Autodesk Inventor part; units mm, degrees
ref_plane "YZ Plane" through (0, 0, 0) normal (1, 0, 0) x (0, 1, 0)
ref_plane "XZ Plane" through (0, 0, 0) normal (0, 1, 0) x (-1, 0, 0)
ref_plane "XY Plane" through (0, 0, 0) normal (0, 0, 1) x (1, 0, 0)
sketch "Sketch1" plane through (0, 0, 0) normal (0, 1, 0) x (-1, 0, 0)
  line L0 (0, 0) -> (28, 0)
  line L1 (28, 0) -> (28, -38.5)
  line L2 (28, -38.5) -> (0, -38.5)
  line L3 (0, -38.5) -> (0, 0)
  dimension "d0" = 28
  dimension "d1" = 38.5
extrude "Extrusion1" add sketch "Sketch1" along normal blind 3
sketch "Sketch2" plane through (0, 3, 0) normal (0, 1, 0) x (1, 0, 0)
  line L0 (-28, 0) -> (0, 0)
  circle A0 centre (0, 0) radius 2
  circle A1 centre (-28, 0) radius 2
  line L1 (0, 38.5) -> (-28, 38.5)
  circle A2 centre (-28, 38.5) radius 2
  circle A3 centre (0, 38.5) radius 2
  dimension "d8" = 4
  dimension "d9" = 4
  dimension "d10" = 4
  dimension "d11" = 4
extrude "Extrusion2" cut sketch "Sketch2" against normal blind 3
sketch "Sketch3" plane through (0, 3, 0) normal (0, 1, 0) x (1, 0, 0)
  line L0 (-32.85, 43.35) -> (4.85, 43.35)
  line L1 (4.85, 43.35) -> (4.85, -4.85)
  line L2 (4.85, -4.85) -> (-32.85, -4.85)
  line L3 (-32.85, -4.85) -> (-32.85, 43.35)
  line L4 (-2, 38.5) -> (-26, 38.5)
  line L5 (0, 2) -> (0, 36.5)
  point P0 (0, 0)
  point P1 (-2, 6.25)
  point P2 (-26, 32.25)
  dimension "d14" = 48.2
  dimension "d15" = 37.7
  dimension "d16" = 4.85
  dimension "d17" = 4.85
extrude "Extrusion3" add sketch "Sketch3" along normal blind 2
sketch "Sketch4" plane through (0, 3, 0) normal (0, -1, 0) x (1, 0, 0)
  circle A0 centre (2.35, -40.85) radius 2.25
  line L0 (-2, -38.5) -> (-26, -38.5)
  line L1 (0, -2) -> (0, -36.5)
  circle A1 centre (-30.35, -40.85) radius 2.25
  line L2 (-28, -36.5) -> (-28, -2)
  circle A2 centre (-30.35, 2.35) radius 2.25
  line L3 (-26, 0) -> (-2, 0)
  circle A3 centre (2.35, 2.35) radius 2.25
  point P0 (0, 0)
  dimension "d20" = 4.5
  dimension "d21" = 2.35
  dimension "d22" = 2.35
  dimension "d23" = 4.5
  dimension "d24" = 2.35
  dimension "d25" = 2.35
  dimension "d26" = 4.5
  dimension "d27" = 2.35
  dimension "d28" = 4.5
  dimension "d29" = 2.35
  dimension "d30" = 2.35
  dimension "d31" = 2.35
extrude "Extrusion4" add sketch "Sketch4" along normal blind 3
fillet "Fillet1" radius 2 4 edges at (4.85, 4, -43.35) (4.85, 4, 4.85) (-32.85, 4, 4.85) (-32.85, 4, -43.35)
sketch "Sketch5" plane through (0, 5, 0) normal (0, 1, 0) x (1, 0, 0)
  circle A0 centre (0, 19.25) radius 1
  circle A1 centre (-28, 19.25) radius 1
  line L0 (4.85, -2.85) -> (4.85, 41.35)
  line L1 (-30.85, -4.85) -> (2.85, -4.85)
  point P0 (0, 0)
  dimension "d45" = 2
  dimension "d46" = 2
  dimension "d73" = 28
  dimension "d81" = 24.1
  dimension "d82" = 4.85
extrude "Extrusion6" cut sketch "Sketch5" against normal through all
sketch "Sketch8" plane through (0, 5, 0) normal (0, 1, 0) x (1, 0, 0)
  circle A0 centre (-14, 3.125) radius 2.5
  line L0 (-2, 6.25) -> (-26, 6.25)
  line L1 (-26, 0) -> (-2, 0)
  line L2 (-32.85, 41.35) -> (-32.85, -2.85)
  point P0 (0, 0)
  dimension "d68" = 5
  dimension "d69" = 3.125
  dimension "d70" = 18.85
extrude "Extrusion9" cut sketch "Sketch8" against normal through all
sketch "Sketch10" plane through (0, 5, 0) normal (0, 1, 0) x (1, 0, 0)
  line L0 (-25.5, 12.75) -> (-2.5, 12.75)
  line L1 (-2.5, 12.75) -> (-2.5, 25.75)
  line L2 (-2.5, 25.75) -> (-25.5, 25.75)
  line L3 (-25.5, 25.75) -> (-25.5, 12.75)
  line L4 (-32.85, 41.35) -> (-32.85, -2.85)
  circle A0 centre (-28, 19.25) radius 1
  point P0 (0, 0)
  dimension "d83" = 23
  dimension "d84" = 13
  dimension "d85" = 7.35
  dimension "d86" = 6.5
extrude "Extrusion11" cut sketch "Sketch10" against normal through all contours L3 L2 L1 L0
sketch "Sketch11" plane through (0, 5, 0) normal (0, 1, 0) x (1, 0, 0)
  line L0 (-32.85, 41.35) -> (-32.85, -2.85)
  line L1 (-32.85, 12.75) -> (4.85, 12.75)
  line L2 (4.85, 12.75) -> (4.85, 43.35)
  line L3 (4.85, 43.35) -> (-32.85, 43.35)
  line L4 (-32.85, 43.35) -> (-32.85, 12.75)
  line L5 (-2.5, 12.75) -> (-25.5, 12.75)
  point P0 (0, 0)
  point P1 (-30.85, 43.35)
  point P2 (4.85, 41.35)
extrude "Extrusion12" cut sketch "Sketch11" against normal through all
sketch "Sketch9" plane through (0, 5, 0) normal (0, 1, 0) x (1, 0, 0)
  circle A0 centre (-14, 3.125) radius 2.5
  line L0 (-15.5, 5.125) -> (-15.5, 12.75)
  line L1 (-15.5, 12.75) -> (-12.5, 12.75)
  line L2 (-12.5, 12.75) -> (-12.5, 5.125)
  arc A1 (-12.5, 5.125) -> (-15.5, 5.125) centre (-14, 3.125) ccw
  line L3 (4.85, 12.75) -> (-32.85, 12.75)
  point P0 (0, 0)
  point P1 (-14, 12.75)
  point P2 (-14, 12.75)
  dimension "d76" = 3
  dimension "d77" = 1.5
extrude "Extrusion13" cut sketch "Sketch9" against normal through all contours A0 L0 L1 L2
fillet "Fillet3" radius 2 2 edges at (-15.5, 2.5, -5.125) (-12.5, 2.5, -5.125)
sketch "Sketch12" plane through (2.35, 0, 2.35) normal (0, -1, 0) x (1, 0, 0)
  point P0 (-2.35, -2.35)
sketch "Sketch13" plane through (0, 5, 0) normal (0, 1, 0) x (1, 0, 0)
  circle A0 centre (2.35, -2.35) radius 2.25
  circle A1 centre (2.35, -2.35) radius 1.15
  circle A2 centre (-30.35, -2.35) radius 2.25
  circle A3 centre (-30.35, -2.35) radius 1.15
  point P0 (0, 0)
  dimension "d96" = 2.3
  dimension "d97" = 2.3
extrude "Extrusion14" cut sketch "Sketch13" against normal through all contours A1 | A3
sketch "Sketch15" plane through (0, 0, -12.75) normal (0, 0, -1) x (-1, 0, 0)
  line L0 (0, 3) -> (-4.85, 3)
  line L1 (30.85, 5) -> (-2.85, 5)
  line L2 (-4.85, 3) -> (2.5, 3)
  line L3 (2.5, 3) -> (2.5, 5)
  line L4 (2.5, 5) -> (-4.85, 5)
  line L5 (-4.85, 5) -> (-4.85, 3)
  line L6 (32.85, 5) -> (32.85, 3)
  line L7 (32.85, 5) -> (25.5, 5)
  line L8 (25.5, 5) -> (25.5, 3)
  line L9 (25.5, 3) -> (32.85, 3)
  line L10 (32.85, 3) -> (32.85, 5)
  point P0 (0, 0)
  point P1 (28, 0)
  dimension "d109" = 2.5
  dimension "d110" = 2.5
extrude "Extrusion16" add sketch "Sketch15" along normal blind 4
sketch "Sketch16" plane through (4.85, 3, 2.85) normal (1, 0, 0) x (0, 0, -1)
  line L0 (19.6, 2) -> (0, 2)
  line L1 (19.6, 0) -> (0, 0)
  line L2 (19.6, 2) -> (19.2, 2)
  line L3 (19.2, 2) -> (19.2, 0)
  line L4 (19.2, 0) -> (19.6, 0)
  line L5 (19.6, 0) -> (19.6, 2)
  point P0 (2.85, -3)
  dimension "d111" = 0.4
extrude "Extrusion17" cut sketch "Sketch16" against normal through all
properties part number "ServoFullMountInsert"
Source: CAD feature listing. Evaluate the final solid. Frame: model axes, mm. A direction names the side the tool comes from. Give positions to 0.01 mm unless a question says otherwise; leave off trailing zeros. Loops run counter-clockwise (first coordinate to the right, second up) from the corner with the lowest first, then second, coordinate; pieces in that order, holes last. Notation, with made-up numbers: (61, 55) - (88, 55) arc R11 ccw to (88, 59) - close; hole circle Ø5 at (-39.75, 40). An arc over 180 degrees is marked (long way). Use CSV: the item, a comma, the result in double quotes. Start each with the question number.
1. Section B-B (z = -11). Output: boundary loops of the cut face in (x, y).
2. Draft query along X for faces 1 (the flat face through (-12.5, 3, -9)), 2 (the cylindrical face through (4.25, 4.01, 4.28)), 3 (the cylindrical face through (-26.57, 1.52, -1.4)), 4 (the cylindrical face through (0.1, 1.5, 2.3)). Return one class per face: +X half, -X half, draft (parallel to the pull), parting line (faces both ways), or undercut.
3. Section A-A (y = 1.25). Output: boundary loops of the cut face in (x, z) (3 decimals).
4. Reachability of faces 5 (the flat face through (-28, 1, -7)), 6 (the flat face through (-14, 1, 0)), 7 (the flat face through (0, 1, -7)), 8 (the cylindrical face through (-12.382, 2.465, -5.278)), 9 (the flat face through (-15.5, 3, -9)) from +Z, -Z, +X, -X, +Y, -Y: full face, straight path, thin tool, end or side. Return the list, or none.
5. Section D-D (y = 3.5). Output: boundary loops of the cut face in (x, z) (3 decimals), then the cut area to 3 significant figures.
6. Ray query, L1, parallel to X at y = 3.35, z = 2.35; L2, parallel to X at y = 2, z = -6; L3, parallel to X at y = 3.25, z = -13.75. Return the intervals inside material, ascending.
7. Pin query (flat end, axial travel): pin 1 (1.5 mm diameter, centred on x = -7.5, y = 2, fed in from -Z); pin 2 (2.5 mm diameter, centred on x = -11.5, y = 1.5, fed in from +Z); pin 3 (1.5 mm diameter, centred on x = -27, z = -0.5, fed in from -Y). Return the tip coordinate at first contact, or that it passes through.
8. Section C-C (z = 2.35). Output: boundary loops of the cut face in (x, y).
Response:
1,outline,"(-32.85, 3) - (-28, 3) - (-28, 0) - (-15.5, 0) - (-15.5, 5) - (-32.85, 5) - close; (-12.5, 0) - (0, 0) - (0, 3) - (4.85, 3) - (4.85, 5) - (-12.5, 5) - close"
2,face 1,"undercut"
2,face 2,"+X half"
2,face 3,"-X half"
2,face 4,"undercut"
3,outline,"circle Ø4.5 at (-30.35, 2.35); (-28, -12.75) - (-15.5, -12.75) - (-15.5, -5.953) arc R2 ccw to (-15.944, -4.696) arc R2.5 cw (long way) to (-12.056, -4.696) arc R2 ccw to (-12.5, -5.953) - (-12.5, -12.75) - (0, -12.75) - (0, -2) arc R2 cw to (-2, 0) - (-26, 0) arc R2 cw to (-28, -2) - close; circle Ø4.5 at (2.35, 2.35); hole circle Ø2.3 at (-30.35, 2.35); hole circle Ø2.3 at (2.35, 2.35)"
4,face 5,"+Z, -Z, -X, -Y"
4,face 6,"+Z, +X, -X, -Y"
4,face 7,"+Z, -Z, +X, -Y"
4,face 8,"+Y, -Y"
4,face 9,"-Z, +Y, -Y"
5,outline,"(-32.85, -16.35) - (-25.5, -16.35) - (-25.5, -12.75) - (-15.5, -12.75) - (-15.5, -5.953) arc R2 ccw to (-15.944, -4.696) arc R2.5 cw (long way) to (-12.056, -4.696) arc R2 ccw to (-12.5, -5.953) - (-12.5, -12.75) - (-2.5, -12.75) - (-2.5, -16.35) - (4.85, -16.35) - (4.85, 2.85) arc R2 ccw to (2.85, 4.85) - (-30.85, 4.85) arc R2 ccw to (-32.85, 2.85) - close; hole circle Ø2.3 at (-30.35, 2.35); hole circle Ø2.3 at (2.35, 2.35)"
5,area,"665 mm²"
6,L1,"-32.85 to -31.5, -29.2 to 1.2, 3.5 to 4.85"
6,L2,"-28 to -15.5, -12.5 to 0"
6,L3,"-32.85 to -25.5, -2.5 to 4.85"
7,pin 1,"z = -12.75"
7,pin 2,"z = 0"
7,pin 3,"y = 3"
8,outline,"(-32.85, 3) - (-32.6, 3) - (-32.6, 0) - (-31.5, 0) - (-31.5, 5) - (-32.85, 5) - close; (-29.2, 0) - (-28.1, 0) - (-28.1, 3) - (0.1, 3) - (0.1, 0) - (1.2, 0) - (1.2, 5) - (-29.2, 5) - close; (3.5, 0) - (4.6, 0) - (4.6, 3) - (4.85, 3) - (4.85, 5) - (3.5, 5) - close"
